Could you check a few things on this model? Use its own coordinates, in mm. A direction names the side the tool comes from. Coordinates: 2 decimals unless noted, no trailing zeros. Loops run counter-clockwise (first coordinate to the right, second up) from the corner with the lowest first, then second, coordinate; pieces in that order, holes last.
1) Will these pins go through, and if not, where does the flat tip stop? P1, Ø6, axis at x = 14, z = 7, coming from the -Y side; P2, Ø10, axis at x = 1, z = 6, coming from the -Y side; P3, Ø5, axis at x = -9, z = -7.5, coming from the -Y side.
2) Imagine slicing it at C-C on y = -9. Please give me the cut outline in (x, z), plus the area to 3 significant figures.
3) For faces 1 (the face through (0, 10, 0)), 2 (the face through (0, 30, -20)), 3 (the face through (0, -18, 12)), which set-ups out of +Z, -Z, +X, -X, +Y, -Y let a thin tool reach every point of the face, with its end or its side?
4) If I drill on line 1 along Y through (x, z) = (-18.35, 0); line 2 along X through (y, z) = (17, -1.5); line 3 along Y through (x, z) = (12, 13), over which ranges is the centre line in solid material (lowest first)?
5) Thinking about a two-plate mould opening in Z: for faces 4 (the face through (9, 60, -14)), 5 (the face through (-14.74, 35.35, -3.27)), 6 (the face through (0, -2, 11)), which applies, released by +Z, released by -Z, zero draft, split by the parting line, or undercut?
6) Imagine slicing it at A-A on y = 40. Please give me the cut outline in (x, z), plus the area to 3 significant figures.
7) Imagine slicing it at D-D on z = 14. Please give me the cut outline in (x, y), plus the area to 3 significant figures.
8) Imagine slicing it at B-B on x = -12.98. Please give me the cut outline in (y, z), plus the area to 3 significant figures.
```python
from build123d import *

# Parameters (mm, degrees)
SKETCH_1_W             = 40
SKETCH_1_H             = 40
EXTRUDE_1_DEPTH        = 60
SKETCH_2_R             = 15.1
CUT_EXTRUDE_1_DEPTH    = 50
SKETCH_3_W             = 40
SKETCH_3_H             = 31
SKETCH_3_R             = 2
EXTRUDE_2_DEPTH        = 8
SKETCH_4_R             = 1.5
CUT_EXTRUDE_2_DEPTH    = 75.833147735
PATTERN_LINEAR_1_COUNT = 2
PATTERN_LINEAR_1_PITCH = 20
FILLET_1_R             = 5


with BuildPart() as part:
    # 草圖1 → 填料-伸長1 (new body)
    with BuildSketch(Plane(origin=(0, 0, 0), x_dir=(1, 0, 0), z_dir=(0, 1, 0))):
        Rectangle(SKETCH_1_W, SKETCH_1_H)
    extrude(amount=EXTRUDE_1_DEPTH)

    # 草圖2 → 除料-伸長1 (cut)
    with BuildSketch(Plane(origin=(0, 60, 0), x_dir=(1, 0, 0), z_dir=(0, 1, 0))):
        with Locations(Location((0, 0, 0), (0, 0, 270))):
            Circle(SKETCH_2_R)
    extrude(amount=-CUT_EXTRUDE_1_DEPTH, mode=Mode.SUBTRACT)

    # 草圖3 → 填料-伸長2 (add)
    with BuildSketch(Plane.XY.offset(20)):
        with Locations((0, -15.5)):
            Rectangle(SKETCH_3_W, SKETCH_3_H)
        with Locations((-12.98, -10.004389258)):
            Circle(SKETCH_3_R, mode=Mode.SUBTRACT)
        with Locations((12.98, -10.004389258)):
            Circle(SKETCH_3_R, mode=Mode.SUBTRACT)
        with Locations((-12.98, -25.004389258)):
            Circle(SKETCH_3_R, mode=Mode.SUBTRACT)
        with Locations((12.98, -25.004389258)):
            Circle(SKETCH_3_R, mode=Mode.SUBTRACT)
    extrude(amount=-EXTRUDE_2_DEPTH)

    # 草圖4 → 除料-伸長2 (cut, through all)
    with BuildSketch(Plane(origin=(20, 0, 0), x_dir=(0, 0, -1), z_dir=(1, 0, 0))):
        with Locations((0, 20)):
            Circle(SKETCH_4_R)
    cut_extrude_2 = extrude(amount=-CUT_EXTRUDE_2_DEPTH, mode=Mode.SUBTRACT)

    # 直線複製排列1: 除料-伸長2 ×2
    with Locations(*[(0, i * PATTERN_LINEAR_1_PITCH, 0) for i in range(1, PATTERN_LINEAR_1_COUNT)]):
        add(cut_extrude_2, mode=Mode.SUBTRACT)

    # 圓角1
    fillet_1_edges = [part.edges().sort_by_distance(p)[0] for p in [
        (-20, -31, 16),
        (0, 0, 12),
        (20, -31, 16),
    ]]
    fillet(fillet_1_edges, radius=FILLET_1_R)


solid = part.part
```
Filled in:
1. P1: stops at y = -1
1. P2: stops at y = -2
1. P3: stops at y = 0
2. outline: (-20, 12) - (-14.71, 12) - (-14.71, 20) - (-20, 20) - close; (-11.25, 12) - (11.25, 12) - (11.25, 20) - (-11.25, 20) - close; (14.71, 12) - (20, 12) - (20, 20) - (14.71, 20) - close
2. area: 265 mm2
3. face 1: +Y
3. face 2: -Z, +X, -X, +Y, -Y
3. face 3: -Z, +X, -X, -Y
4. line 1: y = 0 to 18.5, 21.5 to 38.5, 41.5 to 60
4. line 2: x = -20 to -15.03, 15.03 to 20
4. line 3: y = -31 to -26.75, -23.26 to -11.75, -8.26 to 60
5. face 4: zero draft
5. face 5: undercut
5. face 6: released by -Z
6. outline: (-20, -20) - (20, -20) - (20, -1.5) - (15.03, -1.5) arc R15.1 cw to (-15.03, -1.5) - (-20, -1.5) - close; (-20, 1.5) - (-15.03, 1.5) arc R15.1 cw to (15.03, 1.5) - (20, 1.5) - (20, 20) - (-20, 20) - close
6. area: 854 mm2
7. outline: (-20, -26) arc R5 ccw to (-15, -31) - (15, -31) arc R5 ccw to (20, -26) - (20, 60) - (5.66, 60) - (5.66, 10) - (-5.66, 10) - (-5.66, 60) - (-20, 60) - close; hole circle Ø4 at (-12.98, -25); hole circle Ø4 at (-12.98, -10); hole circle Ø4 at (12.98, -25); hole circle Ø4 at (12.98, -10)
7. area: 3,010 mm2
8. outline: (-31, 12) - (-27, 12) - (-27, 20) - (-31, 20) - close; (-23, 12) - (-12, 12) - (-12, 20) - (-23, 20) - close; (-8, 12) - (-5, 12) arc R5 cw to (0, 7) - (0, -20) - (60, -20) - (60, -7.72) - (10, -7.72) - (10, 7.72) - (60, 7.72) - (60, 20) - (-8, 20) - close
8. area: 1,820 mm2
